The figure shows three views and two pictorial views of one solid part (mm, origin at its lowest corner). Answer the questions. A direction names the side the tool comes from. Give positions to 0.01 mm unless a question says otherwise; leave off trailing zeros. Order: outer loops, then holes, each group sorted by start corner. A loop starts at its lowest first (then second) coordinate and runs counter-clockwise, first axis right, second up. Notation, with made-up numbers: (62.5, 15.5) - (77.5, 15.5) arc R20 cw to (77.5, 25.5) - close; hole circle Ø7 at (79.5, -17). An arc over 180 degrees is marked (long way). Return JSON: item names as keys, results as strings. Group by question number.
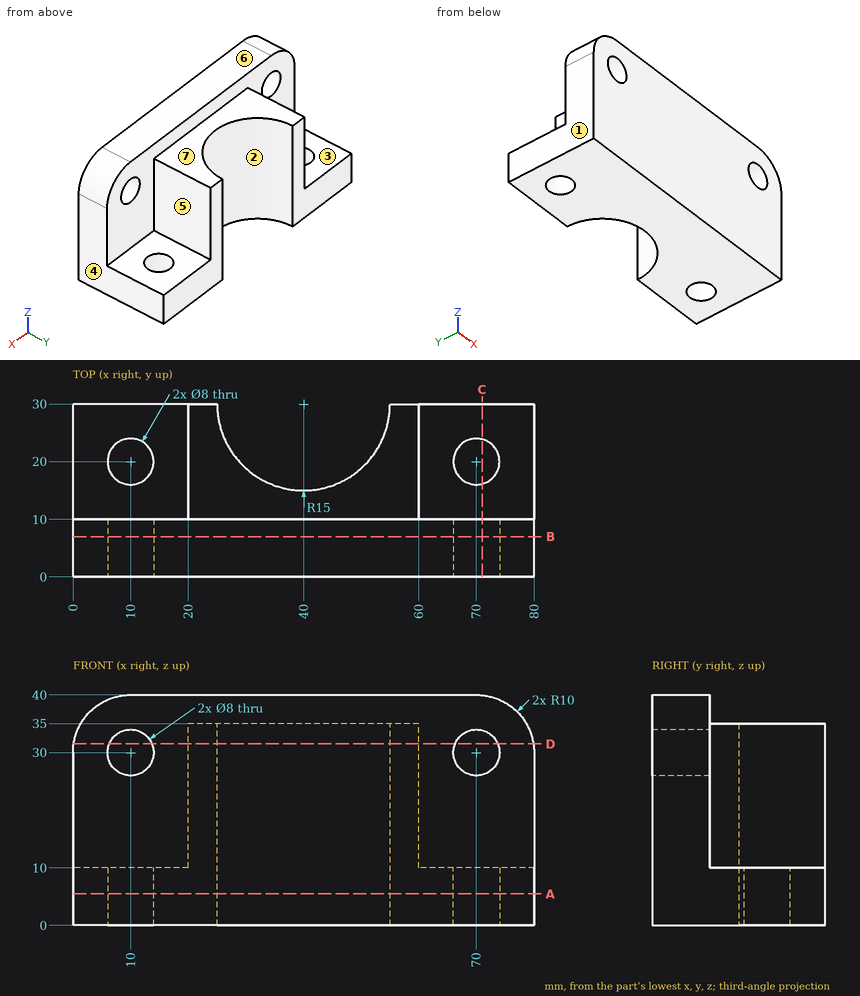
1. Determine the mould class of the marked faces 1, 2, 3 and 4 for opening direction X: released by +X, released by -X, zero draft, split by the parting line, or undercut.
2. Consider probe 1 along X at (y, z) = (2, 30); probe 2 along Y at (x, z) = (70, 4); probe 3 along Y at (x, z) = (9.5, 14.5). Determine where each line is inside the solid, lowest interval first. Write a range as from..to.
3. The part is cut by section B-B (y = 7). Give the vertices of the cut face in (x, z).
4. Each of these flat-tipped pins is pushed along its axis until it touches: pin 1 (12 mm diameter, centred on y = 15.5, z = 25, fed in from +X); pin 2 (6 mm diameter, centred on x = 48.5, y = 23, fed in from +Z); pin 3 (10 mm diameter, centred on y = 24, z = 19, fed in from -X); pin 4 (10.5 mm diameter, centred on x = 10, z = 30, fed in from +Y). Where does it stop, or does it pass through?
5. A tool of negligible diameter and unlimited length cuts with its end or side. For the marked faces 5, 6 and 7, from which of +Z, -Z, +X, -X, +Y, -Y can it reach the whole face along a straight path? Write none if from no direction.
6. The part is cut by section D-D (z = 31.5). Give the vertices of the cut face in (x, y).
7. The part is cut by section A-A (z = 5.5). Give the vertices of the cut face in (x, y).
8. The part is cut by section C-C (x = 71). Give the vertices of the cut face in (y, z).
Answers:
{
 "1": {"face 1": "released by -X", "face 2": "undercut", "face 3": "zero draft", "face 4": "released by +X"},
 "2": {"probe 1": "x = 0..6, 14..66, 74..80", "probe 2": "y = 0..16, 24..30", "probe 3": "y = 0..10"},
 "3": {"outline": "(0, 0) - (80, 0) - (80, 30) arc R10 ccw to (70, 40) - (10, 40) arc R10 ccw to (0, 30) - close; hole circle Ø8 at (10, 30); hole circle Ø8 at (70, 30)"},
 "4": {"pin 1": "stops at x = 80", "pin 2": "passes through", "pin 3": "stops at x = 20", "pin 4": "stops at y = 10"},
 "5": {"face 5": "+Z, +X, +Y", "face 6": "+Z, +X, -X, +Y, -Y", "face 7": "+Z, +X, -X, +Y"},
 "6": {"outline": "(0.11, 0) - (6.29, 0) - (6.29, 10) - (0.11, 10) - close; (13.71, 0) - (66.29, 0) - (66.29, 10) - (60, 10) - (60, 30) - (55, 30) arc R15 cw to (25, 30) - (20, 30) - (20, 10) - (13.71, 10) - close; (73.71, 0) - (79.89, 0) - (79.89, 10) - (73.71, 10) - close"},
 "7": {"outline": "(0, 0) - (80, 0) - (80, 30) - (55, 30) arc R15 cw to (25, 30) - (0, 30) - close; hole circle Ø8 at (10, 20); hole circle Ø8 at (70, 20)"},
 "8": {"outline": "(0, 0) - (16.13, 0) - (16.13, 10) - (10, 10) - (10, 26.13) - (0, 26.13) - close; (0, 33.87) - (10, 33.87) - (10, 39.95) - (0, 39.95) - close; (23.87, 0) - (30, 0) - (30, 10) - (23.87, 10) - close"}
}
